```python
from build123d import *

# Parameters (mm, degrees)
BOSS_EXTRUDE2_DEPTH       = 16.1925
BOSS_EXTRUDE3_DEPTH       = 16.1925
CUT_EXTRUDE1_DEPTH        = 133.157398694
M10_CLEARANCE_SLOT1_DEPTH = 16.1925
CUT_EXTRUDE2_DEPTH        = 9.525
BOSS_EXTRUDE13_DEPTH      = 83.5025
CUT_EXTRUDE6_DEPTH        = 66.548
CUT_EXTRUDE7_DEPTH        = 76.2
CUT_EXTRUDE7_DEPTH_BACK   = 10.16
SKETCH39_R                = 17.78
SKETCH39_R_2              = 19.05
SKETCH40_R                = 7.9375
SKETCH40_R_2              = 9.61898
CUT_EXTRUDE8_DEPTH        = 156.486489701
SKETCH41_R                = 8.89
CUT_EXTRUDE9_DEPTH        = 24.892
SKETCH42_R                = 2.54
SKETCH42_R_2              = 3.81
CUT_EXTRUDE10_DEPTH       = 12.7


# Read off the part's stored shape, not the designer's step: M10 Clearance Slot1
with BuildPart() as part:
    # Sketch2 → Boss-Extrude2 (new body)
    with BuildSketch(Plane.YZ):
        with BuildLine():
            Line((-50.8, -106.3625), (50.8, -106.3625))
            ThreePointArc((50.8, -106.3625), (59.780256121, -102.642756121), (63.5, -93.6625))
            Line((63.5, -93.6625), (63.5, 93.6625))
            ThreePointArc((63.5, 93.6625), (59.780256121, 102.642756121), (50.8, 106.3625))
            Line((50.8, 106.3625), (-50.8, 106.3625))
            ThreePointArc((-50.8, 106.3625), (-59.780256121, 102.642756121), (-63.5, 93.6625))
            Line((-63.5, 93.6625), (-63.5, -93.6625))
            ThreePointArc((-63.5, -93.6625), (-59.780256121, -102.642756121), (-50.8, -106.3625))
        make_face()
    extrude(amount=BOSS_EXTRUDE2_DEPTH)

    # Sketch14 → Boss-Extrude3 (add)
    with BuildSketch(Plane.YZ):
        with BuildLine():
            Line((-63.5, -80.9625), (63.5, -80.9625))
            ThreePointArc((63.5, -80.9625), (69.993196862, 0), (63.5, 80.9625))
            Line((63.5, 80.9625), (-63.5, 80.9625))
            ThreePointArc((-63.5, 80.9625), (-76.748938541, 0), (-63.5, -80.9625))
        make_face()
    extrude(amount=BOSS_EXTRUDE3_DEPTH)

    # Sketch15 → Cut-Extrude1 (cut, through all)
    with BuildSketch(Plane.YZ.offset(16.1925)):
        with BuildLine():
            Line((-38.1, -106.3625), (38.1, -106.3625))
            ThreePointArc((38.1, -106.3625), (29.119743879, -102.642756121), (25.4, -93.6625))
            Line((25.4, -93.6625), (25.4, -80.9625))
            ThreePointArc((25.4, -80.9625), (0, -71.260563314), (-25.4, -80.9625))
            Line((-25.4, -80.9625), (-25.4, -93.6625))
            ThreePointArc((-25.4, -93.6625), (-29.119743879, -102.642756121), (-38.1, -106.3625))
        make_face()
        with BuildLine():
            Line((-38.1, 106.3625), (38.1, 106.3625))
            ThreePointArc((38.1, 106.3625), (29.119743879, 102.642756121), (25.4, 93.6625))
            Line((25.4, 93.6625), (25.4, 80.9625))
            ThreePointArc((25.4, 80.9625), (0, 71.260563314), (-25.4, 80.9625))
            Line((-25.4, 80.9625), (-25.4, 93.6625))
            ThreePointArc((-25.4, 93.6625), (-29.119743879, 102.642756121), (-38.1, 106.3625))
        make_face()
    extrude(amount=-CUT_EXTRUDE1_DEPTH, mode=Mode.SUBTRACT)

    # M10 Clearance Slot1 outline → M10 Clearance Slot1 (cut)
    with BuildSketch(Plane.YZ):
        with BuildLine():
            Line((-38.95, -93.6625), (-38.95, -80.9625))
            ThreePointArc((-38.95, -80.9625), (-44.45, -75.4625), (-49.95, -80.9625))
            Line((-49.95, -80.9625), (-49.95, -93.6625))
            ThreePointArc((-49.95, -93.6625), (-44.45, -99.1625), (-38.95, -93.6625))
        make_face()
        with BuildLine():
            ThreePointArc((-38.95, 93.6625), (-44.45, 99.1625), (-49.95, 93.6625))
            Line((-49.95, 93.6625), (-49.95, 80.9625))
            ThreePointArc((-49.95, 80.9625), (-44.45, 75.4625), (-38.95, 80.9625))
            Line((-38.95, 80.9625), (-38.95, 93.6625))
        make_face()
        with BuildLine():
            Line((49.95, -93.6625), (49.95, -80.9625))
            ThreePointArc((49.95, -80.9625), (44.45, -75.4625), (38.95, -80.9625))
            Line((38.95, -80.9625), (38.95, -93.6625))
            ThreePointArc((38.95, -93.6625), (44.45, -99.1625), (49.95, -93.6625))
        make_face()
        with BuildLine():
            ThreePointArc((49.95, 93.6625), (44.45, 99.1625), (38.95, 93.6625))
            Line((38.95, 93.6625), (38.95, 80.9625))
            ThreePointArc((38.95, 80.9625), (44.45, 75.4625), (49.95, 80.9625))
            Line((49.95, 80.9625), (49.95, 93.6625))
        make_face()
    extrude(amount=M10_CLEARANCE_SLOT1_DEPTH, mode=Mode.SUBTRACT)

    # Sketch31 → Cut-Extrude2 (cut)
    with BuildSketch(Plane.YZ.offset(16.1925)):
        Polygon((-63.5, 106.3625), (63.5, 106.3625), (65.093481902, 106.3625), (65.093481902, 70.385390475), (63.5, 70.385390475), (-63.5, 70.385390475), (-66.802, 70.385390475), (-66.802, 106.3625), align=None)
        Polygon((-63.5, -106.3625), (63.5, -106.3625), (65.03495059, -106.3625), (65.03495059, -70.8025), (63.5, -70.8025), (-63.5, -70.8025), (-66.681318502, -70.8025), (-66.681318502, -106.3625), align=None)
    extrude(amount=-CUT_EXTRUDE2_DEPTH, mode=Mode.SUBTRACT)

    # Sketch35 → Boss-Extrude13 (add)
    with BuildSketch(Plane.YZ.offset(16.1925)):
        with BuildLine():
            Line((-56.656792843, -66.178226808), (1.373429882, -66.178226808))
            ThreePointArc((1.373429882, -66.178226808), (29.681734779, -69.76216524), (57.870185881, -65.333173792))
            ThreePointArc((57.870185881, -65.333173792), (66.517752315, 0.213764908), (57.050540491, 65.647345572))
            ThreePointArc((57.050540491, 65.647345572), (29.463073407, 69.728791712), (1.805161675, 66.155773192))
            Line((1.805161675, 66.155773192), (-56.656792843, 66.155773192))
            Line((-56.656792843, 66.155773192), (-56.656792843, 41.91021734))
            ThreePointArc((-56.656792843, 41.91021734), (-73.855751192, -0.011226808), (-56.656792843, -41.932670956))
            Line((-56.656792843, -41.932670956), (-56.656792843, -66.178226808))
        make_face()
    extrude(amount=BOSS_EXTRUDE13_DEPTH)

    # Sketch38 → Cut-Extrude6 (cut)
    with BuildSketch(Plane.YZ.offset(16.1925)):
        with BuildLine():
            Line((54.087207157, 57.265773192), (54.087207157, -1.408226808))
            ThreePointArc((54.087207157, -1.408226808), (62.460842713, -29.348226808), (54.087207157, -57.288226808))
            ThreePointArc((54.087207157, -57.288226808), (28.687207157, -62.9621542), (3.287207157, -57.288226808))
            Line((3.287207157, -57.288226808), (-47.766792843, -57.288226808))
            Line((-47.766792843, -57.288226808), (-47.766792843, -38.111226808))
            ThreePointArc((-47.766792843, -38.111226808), (-64.965751192, -0.011226808), (-47.766792843, 38.088773192))
            Line((-47.766792843, 38.088773192), (-47.766792843, 57.265773192))
            Line((-47.766792843, 57.265773192), (3.287207157, 57.265773192))
            ThreePointArc((3.287207157, 57.265773192), (28.687207157, 61.623724224), (54.087207157, 57.265773192))
        make_face()
    extrude(amount=CUT_EXTRUDE6_DEPTH, mode=Mode.SUBTRACT)

    # Sketch39 → Cut-Extrude7 (cut, two sides: drawn at the far end of the back side and taken through both)
    with BuildSketch(Plane.YZ.offset(16.1925).offset(-CUT_EXTRUDE7_DEPTH_BACK)):
        with Locations(Location((17.365170467, 39.602870467, 0), (0, 0, 90))):
            Circle(SKETCH39_R)
        with Locations(Location((26.26578479, -28.0035, 0), (0, 0, 90))):
            Circle(SKETCH39_R_2)
        with Locations(Location((-27.0002, 0, 0), (0, 0, 90))):
            Circle(SKETCH39_R)
    extrude(amount=CUT_EXTRUDE7_DEPTH + CUT_EXTRUDE7_DEPTH_BACK, mode=Mode.SUBTRACT)

    # Sketch40 → Cut-Extrude8 (cut, through all)
    with BuildSketch(Plane.YZ.offset(16.1925)):
        with Locations(Location((17.365170467, 39.602870467, 0), (0, 0, 270))):
            Circle(SKETCH40_R)
        with Locations(Location((26.26578479, -28.0035, 0), (0, 0, 270))):
            Circle(SKETCH40_R_2)
    extrude(amount=-CUT_EXTRUDE8_DEPTH, mode=Mode.SUBTRACT)

    # Sketch41 → Cut-Extrude9 (cut)
    with BuildSketch(Plane.YZ.offset(99.695)):
        with Locations(Location((-27.0002, 0, 0), (0, 0, 270))):
            Circle(SKETCH41_R)
    extrude(amount=-CUT_EXTRUDE9_DEPTH, mode=Mode.SUBTRACT)

    # Sketch42 → Cut-Extrude10 (cut, symmetric)
    with BuildSketch(Plane.YZ.offset(16.1925)):
        with Locations(Location((29.681734779, -66.35801684, 0), (0, 0, 270))):
            Circle(SKETCH42_R)
        with Locations(Location((59.416679264, 27.928773192, 0), (0, 0, 270))):
            Circle(SKETCH42_R_2)
        with Locations(Location((29.463073407, 65.674282954, 0), (0, 0, 270))):
            Circle(SKETCH42_R)
        with Locations(Location((-52.211792843, 61.710773192, 0), (0, 0, 270))):
            Circle(SKETCH42_R_2)
        with Locations(Location((-52.211792843, -61.733226808, 0), (0, 0, 270))):
            Circle(SKETCH42_R_2)
    extrude(amount=CUT_EXTRUDE10_DEPTH, both=True, mode=Mode.SUBTRACT)


solid = part.part
```
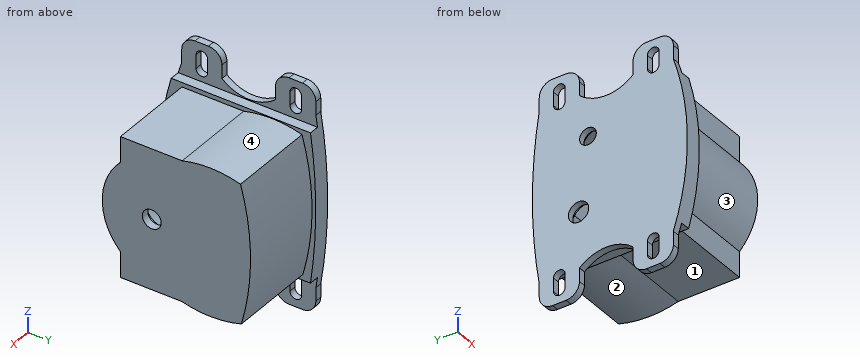
Build history of the part. All positions in model axes, mm. Face numbers are marked on the shaded views. A direction names the side the tool comes from. Give positions to 0.01 mm unless a question says otherwise; leave off trailing zeros. Loops run counter-clockwise (first coordinate to the right, second up) from the corner with the lowest first, then second, coordinate; pieces in that order, holes last. Notation, with made-up numbers: (45, -16) - (65, -16) arc R22 cw to (65, -1) - close; hole circle Ø4 at (-6, 69). An arc over 180 degrees is marked (long way). Use a Markdown table: item, result.
(1) Band-saw the part on B-B (x = 24.5). Give the cut face in (y, z), and give its area (3 significant figures).
Taken from the geometry:
| item | result |
|---|---|
| outline | (-56.66, -66.18) - (1.37, -66.18) arc R101.6 ccw to (57.87, -65.33) arc R241.3 ccw to (57.05, 65.65) arc R101.6 ccw to (1.81, 66.16) - (-56.66, 66.16) - (-56.66, 41.91) arc R59.69 ccw to (-56.66, -41.93) - close; hole circle Ø7.62 at (-52.21, -61.73); hole circle Ø7.62 at (-52.21, 61.71); hole (-47.77, -57.29) - (3.29, -57.29) arc R59.69 ccw to (54.09, -57.29) arc R50.8 ccw to (54.09, -1.41) - (54.09, 57.27) arc R76.2 ccw to (3.29, 57.27) - (-47.77, 57.27) - (-47.77, 38.09) arc R50.8 ccw to (-47.77, -38.11) - close; hole circle Ø5.08 at (29.46, 65.67); hole circle Ø5.08 at (29.68, -66.36); hole circle Ø7.62 at (59.42, 27.93) |
| area | 3,730 mm2 |
(2) Band-saw the part on D-D (y = -32). Give the cut face in (x, z) (1 decimal).
Taken from the geometry:
| item | result |
|---|---|
| outline | (0, -104.8) - (6.7, -104.8) - (6.7, -70.8) - (16.2, -70.8) - (16.2, -66.2) - (99.7, -66.2) - (99.7, -7.4) - (92.4, -7.4) - (92.4, -17.1) - (82.7, -17.1) - (82.7, -57.3) - (16.2, -57.3) - (16.2, -17.1) - (6, -17.1) - (6, 17.1) - (16.2, 17.1) - (16.2, 57.3) - (82.7, 57.3) - (82.7, 17.1) - (92.4, 17.1) - (92.4, 7.4) - (99.7, 7.4) - (99.7, 66.2) - (16.2, 66.2) - (16.2, 70.4) - (6.7, 70.4) - (6.7, 104.8) - (0, 104.8) - close |
(3) Which spindle directions (+Z, -Z, +X, -X, +Y, -Y) get a long thin tool onto all of the face, cutting with end or side? Do the marked faces 1, 2, 3 and 4. Say none if no direction does.
Taken from the geometry:
| item | result |
|---|---|
| face 1 | -Z, +X, -Y |
| face 2 | -Z, +X |
| face 3 | +X, -Y |
| face 4 | +Z, +X |
(4) Drop flat-ended pins along their axis: pin 1 Ø6 at (x, y) = (84, -30.5) entering from -Z; pin 2 Ø5 at (x, y) = (42, 43.5) entering from +Z; pin 3 Ø3 at (x, y) = (59.5, 12) entering from +Z. Give the stop position or say it passes through.
Taken from the geometry:
| item | result |
|---|---|
| pin 1 | z = -66.18 |
| pin 2 | z = 68.96 |
| pin 3 | z = 68.62 |
(5) Band-saw the part on A-A (x = 53). Give the cut face in (y, z).
Taken from the geometry:
| item | result |
|---|---|
| outline | (-56.66, -66.18) - (1.37, -66.18) arc R101.6 ccw to (57.87, -65.33) arc R241.3 ccw to (57.05, 65.65) arc R101.6 ccw to (1.81, 66.16) - (-56.66, 66.16) - (-56.66, 41.91) arc R59.69 ccw to (-56.66, -41.93) - close; hole (-47.77, -57.29) - (3.29, -57.29) arc R59.69 ccw to (54.09, -57.29) arc R50.8 ccw to (54.09, -1.41) - (54.09, 57.27) arc R76.2 ccw to (3.29, 57.27) - (-47.77, 57.27) - (-47.77, 38.09) arc R50.8 ccw to (-47.77, -38.11) - close |
(6) Wall check: line 1 along X through (y, z) = (10, 12) (1 decimal); line 2 along Z through (x, y) = (42, 1.5); line 3 along X through (y, z) = (17.5, 24.5) (1 decimal). Give the ranges that are in metal, low to high.
Taken from the geometry:
| item | result |
|---|---|
| line 1 | 0 to 16.2, 82.7 to 99.7 |
| line 2 | -66.21 to -57.29, 57.27 to 66.16 |
| line 3 | 0 to 6, 92.4 to 99.7 |
(7) Band-saw the part on C-C (z = -28). Give the cut face in (x, y) (1 decimal).
Taken from the geometry:
| item | result |
|---|---|
| outline | (0, -75.2) - (16.2, -75.2) - (16.2, -66.9) - (99.7, -66.9) - (99.7, 65) - (16.2, 65) - (16.2, 69.2) - (0, 69.2) - (0, 35.9) - (6, 35.9) - (6, 45.3) - (16.2, 45.3) - (16.2, 62.4) - (82.7, 62.4) - (82.7, 45.3) - (92.4, 45.3) - (92.4, 7.2) - (82.7, 7.2) - (82.7, -56.6) - (16.2, -56.6) - (16.2, 7.2) - (6, 7.2) - (6, 16.6) - (0, 16.6) - close |
